Geometry: see drawing. Coordinates: mm, zero at the bounding-box minimum. A direction names the side the tool comes from. Give positions to 0.01 mm unless a question says otherwise; leave off trailing zeros. Loops run counter-clockwise (first coordinate to the right, second up) from the corner with the lowest first, then second, coordinate; pieces in that order, holes last. Notation, with made-up numbers: M 82.25,-12 L 136.25,-12 A23 ccw 136.25,-3 Z; hole C 6.5,80 d10. An arc over 180 degrees is marked long. Return JSON: item names as keys, results as strings. Group by question number.
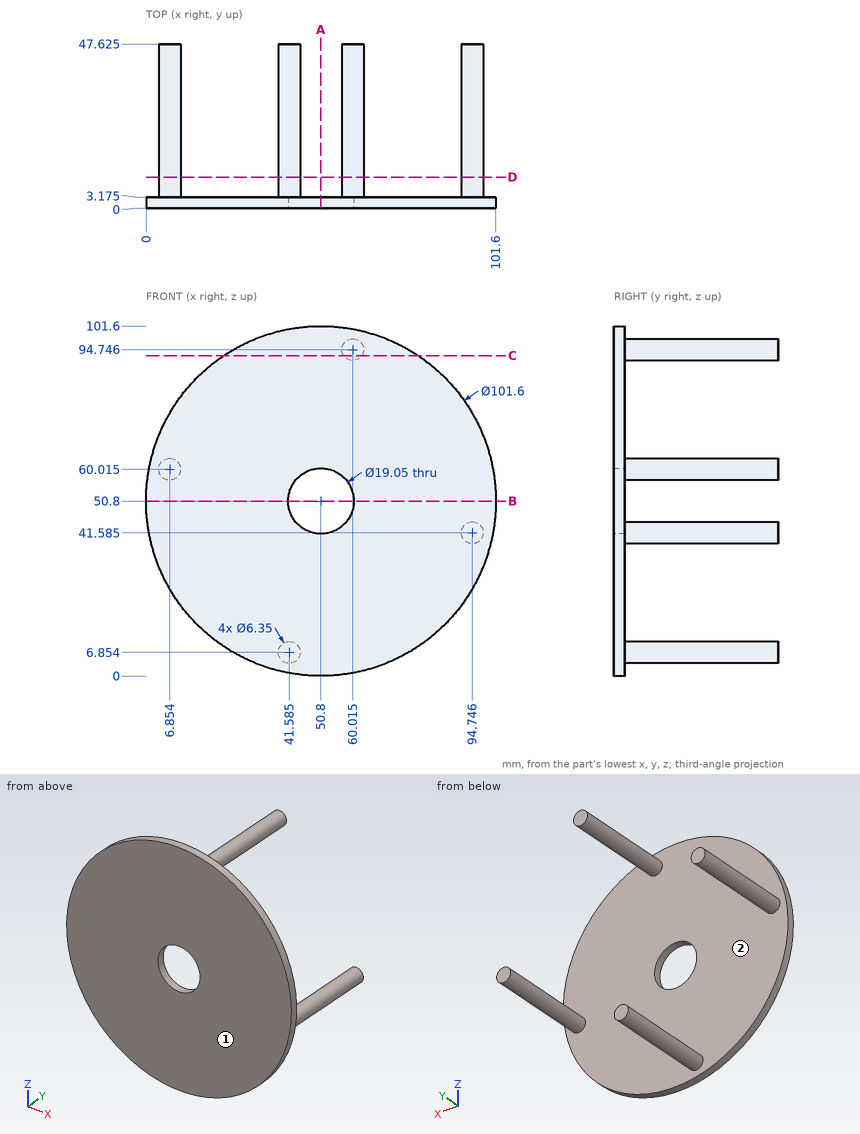
Item 1: Section C-C, the plane z = 93. Return loops of the section in (x, y) (1 decimal).
Item 2: First-contact query: pin 1 Ø3 at (y, z) = (23.5, 40.5) entering from +X; pin 2 Ø5 at (x, y) = (60.5, 26) entering from -Z; pin 3 Ø5 at (x, y) = (60, 17) entering from +Z; pin 4 Ø12 at (x, z) = (82, 12) entering from -Y. Flat tips, straight axial feed; report the tip coordinate or a pass-through.
Item 3: Material intervals for line 1 (Y direction, x = 20, z = 53) (1 decimal); line 2 (X direction, y = 1.4, z = 50.8) (1 decimal); line 3 (X direction, y = 26, z = 41) (1 decimal), sorted ascending. Write a range as from..to.
Item 4: Section A-A, the plane x = 50.8. Return loops of the section in (y, z) (1 decimal), then the cut area to 3 significant figures.
Item 5: Section B-B, the plane z = 50.8. Return loops of the section in (x, y) (1 decimal), then the cut area to 3 significant figures.
Item 6: Section D-D, the plane y = 9. Give the number of separate pieces and of enclosed holes in the cut face, then the cut area to 3 significant figures.
Item 7: Reachability of the marked faces 1 and 2 from +Z, -Z, +X, -X, +Y, -Y: full face, straight path, thin tool, end or side. Return the list, or none.
Answer below:
{
 "1": {"outline": "M 22.5,0 L 79.1,0 L 79.1,3.2 L 62.7,3.2 L 62.7,47.6 L 57.4,47.6 L 57.4,3.2 L 22.5,3.2 Z"},
 "2": {"pin 1": "x = 97.92", "pin 2": "z = 91.57", "pin 3": "z = 97.92", "pin 4": "y = 0"},
 "3": {"line 1": "0..3.2", "line 2": "0..41.3, 60.3..101.6", "line 3": "91.6..97.9"},
 "4": {"outline": "M 0,0 L 3.2,0 L 3.2,41.3 L 0,41.3 Z; M 0,60.3 L 3.2,60.3 L 3.2,101.6 L 0,101.6 Z", "area": "262 mm^2"},
 "5": {"outline": "M 0,0 L 41.3,0 L 41.3,3.2 L 0,3.2 Z; M 60.3,0 L 101.6,0 L 101.6,3.2 L 60.3,3.2 Z", "area": "262 mm^2"},
 "6": {"separate pieces": "4", "enclosed holes": "0", "area": "127 mm^2"},
 "7": {"face 1": "+Z, -Z, +X, -X, -Y", "face 2": "+Y"}
}
